Read the model definition and answer for the solid it produces. Units are mm, in the model's axes. A direction names the side the tool comes from. Give positions to 0.01 mm unless a question says otherwise; leave off trailing zeros. Order: outer loops, then holes, each group sorted by start corner. A loop starts at its lowest first (then second) coordinate and runs counter-clockwise, first axis right, second up. Notation, with made-up numbers: M 1,-25 L 54,-25 A27 ccw 54,13 Z; hole C 2,16.25 d9. An arc over 180 degrees is marked long. One line per item, written item: value.
from build123d import *

# Parameters (mm, degrees)
SKETCH1_W           = 20
SKETCH1_H           = 23
SKETCH1_R           = 0.85
BOSS_EXTRUDE1_DEPTH = 3
SKETCH3_W           = 5
SKETCH3_H           = 3
CUT_EXTRUDE1_DEPTH  = 31.626785662


with BuildPart() as part:
    # Sketch1 → Boss-Extrude1 (new body)
    with BuildSketch(Plane(origin=(0, 0, 0), x_dir=(1, 0, 0), z_dir=(0, 1, 0))):
        with Locations((10, -11.5)):
            Rectangle(SKETCH1_W, SKETCH1_H)
        with Locations(Location((9.886762672, -9.999358845, 0), (0, 0, 270))):
            Circle(SKETCH1_R, mode=Mode.SUBTRACT)
    extrude(amount=BOSS_EXTRUDE1_DEPTH)

    # Sketch3 → Cut-Extrude1 (cut, through all)
    with BuildSketch(Plane(origin=(0, 3, 0), x_dir=(1, 0, 0), z_dir=(0, 1, 0))):
        with Locations((10, -21.5)):
            Rectangle(SKETCH3_W, SKETCH3_H)
    extrude(amount=-CUT_EXTRUDE1_DEPTH, mode=Mode.SUBTRACT)


solid = part.part
1) This flat-tipped pin is pushed along its axis until it touches: pin 1 Ø1.5 at (x, z) = (9.89, 10) entering from +Y. Where does it stop, or does it pass through?
Reported:
pin 1: passes through
2) Find section A-A, the plane z = 9.5. Write down the section's boundary in (x, y), plus the area to 3 significant figures.
Reported:
outline: M 0,0 L 9.2,0 L 9.2,3 L 0,3 Z; M 10.57,0 L 20,0 L 20,3 L 10.57,3 Z
area: 55.9 mm^2
3) Find section C-C, the plane x = 7.75. Write down the section's boundary in (y, z).
Reported:
outline: M 0,0 L 3,0 L 3,20 L 0,20 Z
4) Consider probe 1 along X at (y, z) = (1.7, 21); probe 2 along Z at (x, y) = (11.75, 2.2); probe 3 along Z at (x, y) = (9.25, 0.25). Determine where each line is inside the solid, lowest interval first.
Reported:
probe 1: x = 0 to 7.5, 12.5 to 20
probe 2: z = 0 to 20
probe 3: z = 0 to 9.44, 10.56 to 20
5) Which of the six approach directions +Z, -Z, +X, -X, +Y, -Y give full straight-line access (tool end or side, diameter ignored) to faces 1 (the face through (10, 2, 20)), 2 (the face through (10.46, 1.48, 9.37))?
Reported:
face 1: +Z, +Y, -Y
face 2: +Y, -Y
6) Find section B-B, the plane y = 0.55. Write down the section's boundary in (x, z).
Reported:
outline: M 0,0 L 20,0 L 20,23 L 12.5,23 L 12.5,20 L 7.5,20 L 7.5,23 L 0,23 Z; hole C 9.89,10 d1.7
